Can you work these out from the model? Positions are in its coordinate system, mm. Face numbers are marked on the shaded views. A direction names the side the tool comes from. Round coordinates to 2 decimals unless told otherwise and drop trailing zeros. Loops run counter-clockwise (first coordinate to the right, second up) from the corner with the lowest first, then second, coordinate; pieces in that order, holes last. Notation, with made-up numbers: M -24.75,-21 L -18.75,-21 A16 cw -18.75,-3 Z; hole C -15.75,46.5 d7. An arc over 180 degrees is marked long. Return JSON: item names as keys, results as strings.
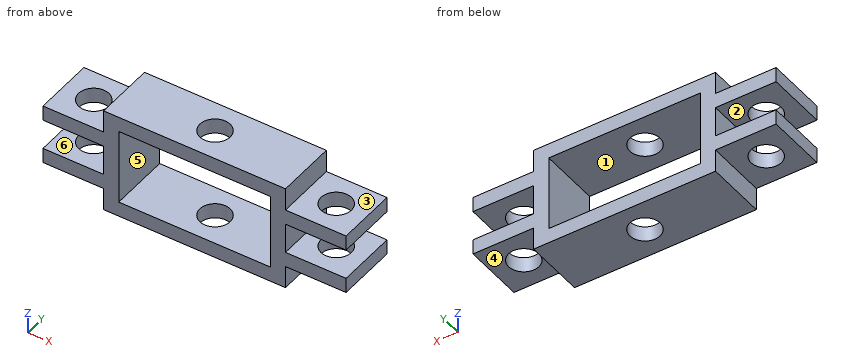
```python
from build123d import *

# Parameters (mm, degrees)
SKETCH2_W           = 60
SKETCH2_H           = 35
SKETCH2_W_2         = 50
SKETCH2_H_2         = 25
BOSS_EXTRUDE1_DEPTH = 20
SKETCH3_R           = 5
CUT_EXTRUDE1_DEPTH  = 36
SKETCH4_W           = 20
SKETCH4_H           = 20
BOSS_EXTRUDE2_DEPTH = 20
SKETCH5_W           = 20
SKETCH5_H           = 20
BOSS_EXTRUDE3_DEPTH = 20
SKETCH6_R           = 5
CUT_EXTRUDE2_DEPTH  = 28.5
SKETCH7_W           = 20
SKETCH7_H           = 10
CUT_EXTRUDE3_DEPTH  = 21


with BuildPart() as part:
    # Sketch2 → Boss-Extrude1 (new body)
    with BuildSketch(Plane(origin=(0, 0, 0), x_dir=(1, 0, 0), z_dir=(0, 1, 0))):
        Rectangle(SKETCH2_W, SKETCH2_H)
        Rectangle(SKETCH2_W_2, SKETCH2_H_2, mode=Mode.SUBTRACT)
    extrude(amount=BOSS_EXTRUDE1_DEPTH)

    # Sketch3 → Cut-Extrude1 (cut, through all)
    with BuildSketch(Plane.XY.offset(17.5)):
        with Locations((0, 10)):
            Circle(SKETCH3_R)
    extrude(amount=-CUT_EXTRUDE1_DEPTH, mode=Mode.SUBTRACT)

    # Sketch4 → Boss-Extrude2 (add)
    with BuildSketch(Plane.ZY.offset(30)):
        with Locations((0, 10)):
            Rectangle(SKETCH4_W, SKETCH4_H)
    extrude(amount=BOSS_EXTRUDE2_DEPTH)

    # Sketch5 → Boss-Extrude3 (add)
    with BuildSketch(Plane(origin=(30, 0, 0), x_dir=(0, 0, -1), z_dir=(1, 0, 0))):
        with Locations((0, 10)):
            Rectangle(SKETCH5_W, SKETCH5_H)
    extrude(amount=BOSS_EXTRUDE3_DEPTH)

    # Sketch6 → Cut-Extrude2 (cut, through all)
    with BuildSketch(Plane.XY.offset(10)):
        with Locations((-40, 10)):
            Circle(SKETCH6_R)
        with Locations((40, 10)):
            Circle(SKETCH6_R)
    extrude(amount=-CUT_EXTRUDE2_DEPTH, mode=Mode.SUBTRACT)

    # Sketch7 → Cut-Extrude3 (cut, through all)
    with BuildSketch(Plane(origin=(0, 20, 0), x_dir=(1, 0, 0), z_dir=(0, 1, 0))):
        with Locations((40, 0)):
            Rectangle(SKETCH7_W, SKETCH7_H)
        with Locations((-40, 0)):
            Rectangle(SKETCH7_W, SKETCH7_H)
    extrude(amount=-CUT_EXTRUDE3_DEPTH, mode=Mode.SUBTRACT)


solid = part.part
```
Q1. Thinking about a two-plate mould opening in X: for the marked faces 5 and 6, which applies, pulls with the +X half, pulls with the -X half, needs draft (parallel to the pull), parting line crosses it, or undercut?
Results:
{"face 5": "undercut", "face 6": "needs draft"}
Q2. I'm going to push flat-ended pins straight in: pin 1 Ø9 at (x, y) = (0, 10) entering from +Z; pin 2 Ø8 at (y, z) = (11, -12) entering from +X; pin 3 Ø1 at (y, z) = (2.5, 3.5) entering from -X; pin 4 Ø6 at (y, z) = (7.5, 14) entering from +X. Where does each tip first touch, or does it pass through?
Results:
{"pin 1": "passes through", "pin 2": "stops at x = 50", "pin 3": "stops at x = -30", "pin 4": "stops at x = 30"}
Q3. If I drill on line 1 along X through (y, z) = (17, 3); line 2 along Z through (x, y) = (-18, 4.5); line 3 along Y through (x, z) = (0, -14.5), over which ranges is the centre line in solid material (lowest first)?
Results:
{"line 1": "x = -30 to -25, 25 to 30", "line 2": "z = -17.5 to -12.5, 12.5 to 17.5", "line 3": "y = 0 to 5, 15 to 20"}
Q4. Suppose I cut it at D-D, the plane y = 7. State how many separate pieces and enclosed holes the cut face has, plus the area to 3 significant figures.
Results:
{"separate pieces": "6", "enclosed holes": "0", "area": "1,010 mm2"}
Q5. Suppose I cut it at C-C, the plane x = 4. Please give me the cut outline in (y, z), plus the area to 3 significant figures.
Results:
{"outline": "M 0,-17.5 L 7,-17.5 L 7,-12.5 L 0,-12.5 Z; M 0,12.5 L 7,12.5 L 7,17.5 L 0,17.5 Z; M 13,-17.5 L 20,-17.5 L 20,-12.5 L 13,-12.5 Z; M 13,12.5 L 20,12.5 L 20,17.5 L 13,17.5 Z", "area": "140 mm2"}
Q6. Suppose I cut it at A-A, the plane y = 1.5. Please give me the cut outline in (x, z).
Results:
{"outline": "M -50,-10 L -30,-10 L -30,-17.5 L 30,-17.5 L 30,-10 L 50,-10 L 50,-5 L 30,-5 L 30,5 L 50,5 L 50,10 L 30,10 L 30,17.5 L -30,17.5 L -30,10 L -50,10 L -50,5 L -30,5 L -30,-5 L -50,-5 Z; hole M -25,-12.5 L 25,-12.5 L 25,12.5 L -25,12.5 Z"}
Q7. On a 3-axis mill with a long thin cutter (end or side, diameter ignored), from which of +Z, -Z, +X, -X, +Y, -Y can I reach the whole of each face in a straight line? I mean the marked faces 1, 2, 3 and 4. Say none if no direction works.
Results:
{"face 1": "+Y, -Y", "face 2": "-X, +Y, -Y", "face 3": "+Z, +X, +Y, -Y", "face 4": "-Z, +X, +Y, -Y"}
Q8. Suppose I cut it at B-B, the plane z = 8. Please give me the cut outline in (x, y), plus the area to 3 significant figures.
Results:
{"outline": "M -50,0 L -25,0 L -25,20 L -50,20 Z; M 25,0 L 50,0 L 50,20 L 25,20 Z; hole C -40,10 d10; hole C 40,10 d10", "area": "843 mm2"}
